The listing builds one solid part. Answer for the finished solid, in the listing's coordinates (mm). Face numbers are marked on the shaded views. A direction names the side the tool comes from. Coordinates: 2 decimals unless noted, no trailing zeros. Write each loop counter-clockwise with the first axis right and the second up, starting at its lowest first coordinate (ties: lowest second). Pieces come first, ordered by that corner, then holes. Notation, with made-up numbers: M 46.5,39.25 L 59.5,39.25 A33 cw 59.5,78.25 Z; hole C -16,14.5 d5. An arc over 180 degrees is marked long. Answer as CSV lines item,"result".
```python
from build123d import *

# Parameters (mm, degrees)
F0_R     = 3.800771
F1_DEPTH = 50.8
F3_D     = 6.35
F2_R     = 14.830071
F2_R_2   = 15.542538
F4_DEPTH = 50.8
F6_DEPTH = 25.4
F8_D     = 6.35
F9_D     = 6.35


with BuildPart() as f1:
    # F0 (on Front) → F1 (new body)
    with BuildSketch(Plane.XZ):
        with BuildLine():
            Line((-17.417282, 46.986144), (-79.371665, 46.986144))
            ThreePointArc((-79.371665, 46.986144), (-93.436013, 41.160501), (-99.261656, 27.096153))
            Line((-99.261656, 27.096153), (-99.261656, -52.813884))
            Line((-99.261656, -52.813884), (72.118267, -52.813884))
            Line((72.118267, -52.813884), (72.118267, -42.549405))
            ThreePointArc((72.118267, -42.549405), (45.893912, 20.761789), (-17.417282, 46.986144))
        make_face()
        with Locations((17.000813, 29.867163)):
            Circle(F0_R, mode=Mode.SUBTRACT)
    extrude(amount=F1_DEPTH)

    # F3 (through all)
    with Locations(Plane.XZ.offset(50.8)):
        with Locations((-78.307003, -42.858165), (35.819549, -42.858165)):
            Hole(F3_D / 2)

    # F2 (on face) → F4 (cut)
    with BuildSketch(Plane.XZ.offset(50.8)):
        with Locations((-78.307003, -42.858165)):
            Circle(F2_R)
        with Locations((35.819549, -42.858165)):
            Circle(F2_R_2)
    extrude(amount=-F4_DEPTH, mode=Mode.SUBTRACT)

    # F5 (on face) → F6 (join)
    with BuildSketch(Plane(origin=(0, 0, -52.813884), x_dir=(1, 0, 0), z_dir=(0, 0, -1))):
        Polygon((23.884133, 22.274217), (23.884133, 18.090272), (23.884133, 13.775429), (55.002525, 13.775429), (55.002525, 37.086386), (23.884133, 37.086386), (23.884133, 35.816312), align=None)
        Polygon((9.837548, 22.274217), (23.884133, 22.274217), (23.884133, 35.816312), (23.884133, 37.086386), (9.837548, 37.086386), align=None)
        Polygon((23.884133, 13.775429), (23.884133, 18.090272), (23.884133, 22.274217), (9.837548, 22.274217), (9.837548, 13.775429), align=None)
        Polygon((-67.315431, 17.847452), (-67.315431, 13.775429), (-54.996047, 13.775429), (-54.996047, 37.086386), (-67.315431, 37.086386), (-67.315431, 35.087846), align=None)
        Polygon((-96.761517, 13.775429), (-67.315431, 13.775429), (-67.315431, 17.847452), (-67.315431, 35.087846), (-67.315431, 37.086386), (-96.761517, 37.086386), align=None)
    extrude(amount=-F6_DEPTH)

    # F8 (through all)
    with Locations(Plane(origin=(0, -13.775429, 0), x_dir=(-1, 0, 0), z_dir=(0, 1, 0))):
        with Locations((-35.819549, -42.858165)):
            Hole(F8_D / 2)

    # F9 (through all)
    with Locations(Plane(origin=(0, -13.775429, 0), x_dir=(-1, 0, 0), z_dir=(0, 1, 0))):
        with Locations((78.064188, -42.372521)):
            Hole(F9_D / 2)


solid = f1.part
```
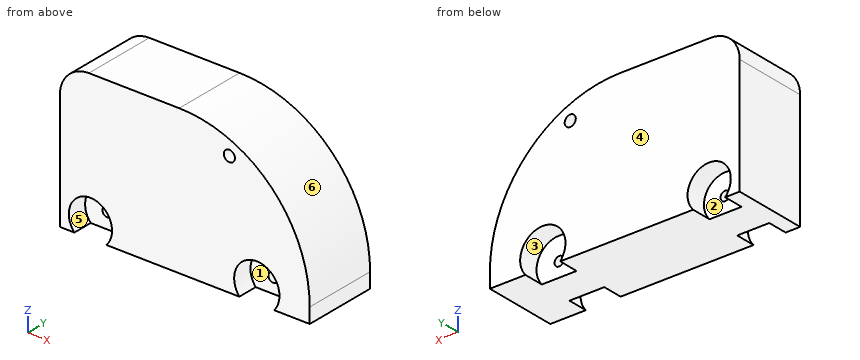
Q1. For the marked faces 1, 2 and 3, determine the directions among +Z, -Z, +X, -X, +Y, -Y from which every point of the face is accessible in a straight line to the end or side of a thin tool.
Output:
face 1,"-Y"
face 2,"+Y"
face 3,"none"
Q2. Find section B-B (y = -3.5). Give the vertices of the cut face in (x, z).
Output:
outline,"M -99.26,-52.81 L -89.3,-52.81 A14.83 cw long -67.32,-52.81 L 23.88,-52.81 A15.54 cw long 47.75,-52.81 L 72.12,-52.81 L 72.12,-42.55 A89.54 ccw -17.42,46.99 L -79.37,46.99 A19.89 ccw -99.26,27.1 Z; hole C 17,29.87 d7.6"
Q3. Flat-ended cylindrical pins translate along their axes: pin 1 Ø8.5 at (x, z) = (35.82, -42.86) entering from -Y; pin 2 Ø7.5 at (x, z) = (-82.5, -38.5) entering from +Y; pin 3 Ø1.7 at (x, y) = (35, -22.5) entering from +Z. Find the tip coordinate at first contact, or state that the pin passes through.
Output:
pin 1,"y = -37.09"
pin 2,"y = -13.78"
pin 3,"z = 30.65"
Q4. Straight lines are drawn through the part: line 1 (X direction, y = -11.5, z = -42); line 2 (X direction, y = -40.5, z = -39); line 3 (X direction, y = -11, z = 30). For each, find the intervals that lie inside material, in ascending order.
Output:
line 1,"-99.26 to -93.11, -63.5 to 20.3, 51.34 to 72.12"
line 2,"-99.26 to -92.63, -63.99 to 20.76, 50.88 to 72.05"
line 3,"-99.05 to 13.2, 20.8 to 35.05"
Q5. Find section D-D (x = 10). Give the vertices of the cut face in (y, z), and give its area (3 significant figures).
Output:
outline,"M -50.8,-52.81 L 0,-52.81 L 0,42.69 L -50.8,42.69 Z"
area,"4,850 mm2"
Q6. Find section C-C (z = -30.5). Give the vertices of the cut face in (x, y).
Output:
outline,"M -99.26,-50.8 L -86.5,-50.8 L -86.5,-37.09 L -70.11,-37.09 L -70.11,-50.8 L 26.39,-50.8 L 26.39,-37.09 L 45.25,-37.09 L 45.25,-50.8 L 71.3,-50.8 L 71.3,0 L 45.25,0 L 45.25,-13.78 L 26.39,-13.78 L 26.39,0 L -70.11,0 L -70.11,-13.78 L -86.5,-13.78 L -86.5,0 L -99.26,0 Z"
Q7. Find section A-A (y = -24). Give the vertices of the cut face in (x, z) (3 decimals).
Output:
outline,"M -99.262,-52.814 L 72.118,-52.814 L 72.118,-42.549 A89.536 ccw -17.417,46.986 L -79.372,46.986 A19.89 ccw -99.262,27.096 Z; hole C -78.064,-42.373 d6.35; hole C 17.001,29.867 d7.602; hole C 35.82,-42.858 d6.35; hole M 34.075,-27.414 L 37.564,-27.414 A15.543 ccw Z"
Q8. The mould has two halves that part along Z. Classify the marked faces 4, 5 and 6: pulls with the +Z half, pulls with the -Z half, needs draft (parallel to the pull), parting line crosses it, or undercut.
Output:
face 4,"needs draft"
face 5,"undercut"
face 6,"pulls with the +Z half"
